```python
from build123d import *

# Parameters (mm, degrees)
SKETCH_1_R          = 40
EXTRUDE_1_DEPTH     = 37.4
CUT_EXTRUDE_1_DEPTH = 16.7
SKETCH_3_R          = 25
CUT_EXTRUDE_2_DEPTH = 6.45
SKETCH_4_R          = 1.5
CUT_EXTRUDE_3_DEPTH = 61.236948794


with BuildPart() as part:
    # 草图1 → 凸台-拉伸1 (new body)
    with BuildSketch(Plane(origin=(0, 0, 0), x_dir=(1, 0, 0), z_dir=(0, 1, 0))):
        with Locations(Location((0, 0, 0), (0, 0, 270))):
            Circle(SKETCH_1_R)
    extrude(amount=EXTRUDE_1_DEPTH)

    # 草图2 → 切除-拉伸1 (cut)
    with BuildSketch(Plane(origin=(0, 37.4, 0), x_dir=(1, 0, 0), z_dir=(0, 1, 0))):
        Polygon((3.493353, 1.52200027), (0.428585602, 3.786332577), (-3.064767398, 2.264332307), (-3.493353, -1.52200027), (-0.428585602, -3.786332577), (3.064767398, -2.264332307), align=None)
    cut_extrude_1 = extrude(amount=-CUT_EXTRUDE_1_DEPTH, mode=Mode.SUBTRACT)

    # 草图3 → 切除-拉伸2 (cut)
    with BuildSketch(Plane(origin=(0, 37.4, 0), x_dir=(1, 0, 0), z_dir=(0, 1, 0))):
        with Locations(Location((0, 0, 0), (0, 0, 270))):
            Circle(SKETCH_3_R)
    cut_extrude_2 = extrude(amount=-CUT_EXTRUDE_2_DEPTH, mode=Mode.SUBTRACT)

    # 草图4 → 切除-拉伸3 (cut, through all)
    with BuildSketch(Plane(origin=(0, 20.7, 0), x_dir=(1, 0, 0), z_dir=(0, 1, 0))):
        with Locations(Location((0, 0, 0), (0, 0, 270))):
            Circle(SKETCH_4_R)
    extrude(amount=-CUT_EXTRUDE_3_DEPTH, mode=Mode.SUBTRACT)

    # 镜向3: 切除-拉伸1, 切除-拉伸2 across plane
    add(cut_extrude_1.mirror(Plane.ZX.offset(18.7)), mode=Mode.SUBTRACT)
    add(cut_extrude_2.mirror(Plane.ZX.offset(18.7)), mode=Mode.SUBTRACT)


solid = part.part
```
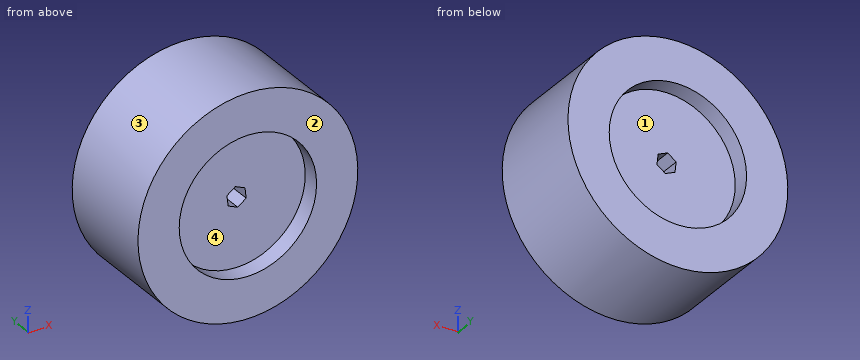
Work out the finished part from the listing and answer in its coordinate system (mm). Face numbers are marked on the shaded views. Round coordinates to 2 decimals unless told otherwise and drop trailing zeros. Order: outer loops, then holes, each group sorted by start corner. A loop starts at its lowest first (then second) coordinate and runs counter-clockwise, first axis right, second up.
Q1. A cutting plane is placed at B-B, the plane z = 0. Determine the outline of the cut face in (x, y), then the cut area to 3 significant figures.
Solution:
outline: (-40, 0) - (-25, 0) - (-25, 6.45) - (-3.32, 6.45) - (-3.32, 16.7) - (-1.5, 16.7) - (-1.5, 20.7) - (-3.32, 20.7) - (-3.32, 30.95) - (-25, 30.95) - (-25, 37.4) - (-40, 37.4) - close; (1.5, 16.7) - (3.32, 16.7) - (3.32, 6.45) - (25, 6.45) - (25, 0) - (40, 0) - (40, 37.4) - (25, 37.4) - (25, 30.95) - (3.32, 30.95) - (3.32, 20.7) - (1.5, 20.7) - close
area: 2,200 mm2
Q2. A cutting plane is placed at C-C, the plane x = -12. Determine the outline of the cut face in (y, z).
Solution:
outline: (0, -38.16) - (37.4, -38.16) - (37.4, -21.93) - (30.95, -21.93) - (30.95, 21.93) - (37.4, 21.93) - (37.4, 38.16) - (0, 38.16) - (0, 21.93) - (6.45, 21.93) - (6.45, -21.93) - (0, -21.93) - close
Q3. Find the intervals of material crossed by line 1 along X through (y, z) = (2, 0); line 2 along X through (y, z) = (17.85, 0); line 3 along Y through (x, z) = (-2, 19), in increasing order.
Solution:
line 1: x = -40 to -25, 25 to 40
line 2: x = -40 to -1.5, 1.5 to 40
line 3: y = 6.45 to 30.95
Q4. The mould has two halves that part along Z. Classify the marked faces 1, 2, 3 and 4: pulls with the +Z half, pulls with the -Z half, needs draft (parallel to the pull), parting line crosses it, or undercut.
Solution:
face 1: undercut
face 2: needs draft
face 3: parting line crosses it
face 4: undercut
Q5. Given pin 1 Ø4 at (x, z) = (-9.5, -3.5) entering from -Y; pin 2 Ø3 at (x, y) = (28, 18) entering from -Z; pin 3 Ø3 at (y, z) = (32, 9) entering from -X; pin 4 Ø1.8 at (x, z) = (0, 0) entering from +Y, each flat-ended and moving along its own axis, determine where each tip first touches the part or whether it passes through.
Solution:
pin 1: stops at y = 6.45
pin 2: stops at z = -29.96
pin 3: stops at x = -39.29
pin 4: passes through
Q6. A cutting plane is placed at A-A, the plane y = 14. Determine the outline of the cut face in (x, z), then the cut area to 3 significant figures.
Solution:
outline: circle Ø80 at (0, 0); hole (-3.49, 1.52) - (-3.06, -2.26) - (0.43, -3.79) - (3.49, -1.52) - (3.06, 2.26) - (-0.43, 3.79) - close
area: 4,990 mm2
Q7. A cutting plane is placed at D-D, the plane z = 14. Determine the outline of the cut face in (x, y), then the cut area to 3 significant figures.
Solution:
outline: (-37.47, 0) - (-20.71, 0) - (-20.71, 6.45) - (20.71, 6.45) - (20.71, 0) - (37.47, 0) - (37.47, 37.4) - (20.71, 37.4) - (20.71, 30.95) - (-20.71, 30.95) - (-20.71, 37.4) - (-37.47, 37.4) - close
area: 2,270 mm2
